```python
from build123d import *

# Parameters (mm, degrees)
BOSS_EXTRUDE1_DEPTH = 86.106
SKETCH2_R           = 2.38125
CUT_EXTRUDE1_DEPTH  = 1.778
SKETCH3_R           = 2.38125
CUT_EXTRUDE2_DEPTH  = 1.778


with BuildPart() as part:
    # Sketch1 → Boss-Extrude1 (new body)
    with BuildSketch(Plane(origin=(0, 0, 0), x_dir=(1, 0, 0), z_dir=(0, 1, 0))):
        Polygon((0, 0), (0, 19.05), (-19.05, 19.05), (-19.05, 17.272), (-1.778, 17.272), (-1.778, 0), align=None)
    extrude(amount=BOSS_EXTRUDE1_DEPTH)

    # Sketch2 → Cut-Extrude1 (cut)
    with BuildSketch(Plane.ZY.offset(1.778)):
        with Locations((-9.525, 76.581)):
            Circle(SKETCH2_R)
        with Locations((-9.525, 9.525)):
            Circle(SKETCH2_R)
    extrude(amount=-CUT_EXTRUDE1_DEPTH, mode=Mode.SUBTRACT)

    # Sketch3 → Cut-Extrude2 (cut)
    with BuildSketch(Plane.XY.offset(-17.272)):
        with Locations((-9.525, 9.525)):
            Circle(SKETCH3_R)
        with Locations((-9.525, 76.581)):
            Circle(SKETCH3_R)
    extrude(amount=-CUT_EXTRUDE2_DEPTH, mode=Mode.SUBTRACT)


solid = part.part
```
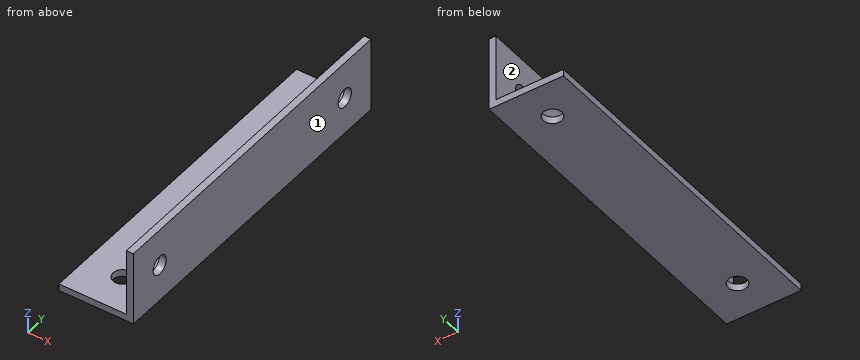
Build history of the part. All positions in model axes, mm. Face numbers are marked on the shaded views. A direction names the side the tool comes from. Give positions to 0.01 mm unless a question says otherwise; leave off trailing zeros. Loops run counter-clockwise (first coordinate to the right, second up) from the corner with the lowest first, then second, coordinate; pieces in that order, holes last. Notation, with made-up numbers: (49, 62.5) -> (90, 62.5) arc R24 cw to (90, 97.5) -> close; hole circle Ø9 at (23, 18). An arc over 180 degrees is marked (long way). One line per question, with ' | ' between items. Start each with the question number.
1) 3-axis set-ups, long thin cutter, end or side, ignore diameter. For the marked faces 1 and 2: which of +Z, -Z, +X, -X, +Y, -Y reach the whole face in a straight line?
2) Cut at A-A (x = -8). Give the cut face in (y, z).
3) Cut at B-B (z = -10.75). Give the cut face in (x, y).
4) Pin check, flat tips, straight feed: pin 1 (10 mm diameter, centred on y = 73, z = -16, fed in from +X); pin 2 (5.5 mm diameter, centred on y = 9.525, z = -9.525, fed in from -X); pin 3 (6 mm diameter, centred on x = -9.525, y = 76.581, fed in from +Z). Stop position of each tip, or through.
5) Probe L1, parallel to Y at x = -11, z = -17.75; L2, parallel to Z at x = -15, y = 62.5; L3, parallel to X at y = 11.5, z = -7.5. List the from-to ranges inside material, lowest first.
6) Cut at C-C (y = 58). Give the cut face in (x, z).
Return value:
1) face 1: +Z, -Z, +X, +Y, -Y | face 2: +Z, -X, +Y, -Y
2) outline: (0, -19.05) -> (7.7, -19.05) -> (7.7, -17.27) -> (0, -17.27) -> close; (11.35, -19.05) -> (74.75, -19.05) -> (74.75, -17.27) -> (11.35, -17.27) -> close; (78.41, -19.05) -> (86.11, -19.05) -> (86.11, -17.27) -> (78.41, -17.27) -> close
3) outline: (-1.78, 0) -> (0, 0) -> (0, 7.48) -> (-1.78, 7.48) -> close; (-1.78, 11.57) -> (0, 11.57) -> (0, 74.54) -> (-1.78, 74.54) -> close; (-1.78, 78.62) -> (0, 78.62) -> (0, 86.11) -> (-1.78, 86.11) -> close
4) pin 1: x = 0 | pin 2: x = -1.78 | pin 3: z = -17.27
5) L1: 0 to 7.66, 11.39 to 74.71, 78.45 to 86.11 | L2: -19.05 to -17.27 | L3: -1.78 to 0
6) outline: (-19.05, -19.05) -> (0, -19.05) -> (0, 0) -> (-1.78, 0) -> (-1.78, -17.27) -> (-19.05, -17.27) -> close
